Design review of the part built by this model. Coordinates are the model's own, in mm. Face numbers are marked on the shaded views. Give positions to 0.01 mm unless a question says otherwise; leave off trailing zeros. Write each loop counter-clockwise with the first axis right and the second up, starting at its lowest first coordinate (ties: lowest second). Pieces come first, ordered by that corner, then holes. Notation, with made-up numbers: M 63,4.5 L 113,4.5 A23 cw 113,22.5 Z; hole C 64.25,33 d2. An arc over 180 degrees is marked long. Use one line per item in the form item = value. Start each with the question number.
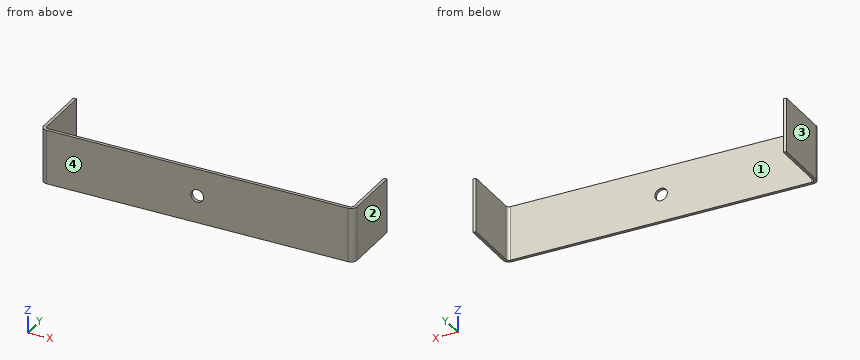
from build123d import *

# Parameters (mm, degrees)
SM_BASE_FLANGE_1_DEPTH = 6.5
OTHER_1_OUTLINE_R      = 1.5
OTHER_1_DEPTH          = 0.7366


# Read off the part's stored shape, not the designer's step: Отверстие1
# Sheet-metal steps are written as plain solids
with BuildPart() as part:
    # Sketch 1 → Базовая кромка1 (new, symmetric)
    with BuildSketch(Plane.XY):
        with BuildLine():
            Line((-37.5, 15), (-37.5, 1.4732))
            ThreePointArc((-37.5, 1.4732), (-37.06850971, 0.43149029), (-36.0268, 0))
            Line((-36.0268, 0), (36.0268, 0))
            ThreePointArc((36.0268, 0), (37.06850971, 0.43149029), (37.5, 1.4732))
            Line((37.5, 1.4732), (37.5, 15))
            Line((37.5, 15), (36.7634, 15))
            Line((36.7634, 15), (36.7634, 1.4732))
            ThreePointArc((36.7634, 1.4732), (36.547654855, 0.952345145), (36.0268, 0.7366))
            Line((36.0268, 0.7366), (-36.0268, 0.7366))
            ThreePointArc((-36.0268, 0.7366), (-36.547654855, 0.952345145), (-36.7634, 1.4732))
            Line((-36.7634, 1.4732), (-36.7634, 15))
            Line((-36.7634, 15), (-37.5, 15))
        make_face()
    extrude(amount=SM_BASE_FLANGE_1_DEPTH, both=True)

    # Отверстие1 outline → Отверстие1 (cut)
    with BuildSketch(Plane(origin=(0, 0, 0), x_dir=(1, 0, 0), z_dir=(0, 1, 0))):
        Circle(OTHER_1_OUTLINE_R)
    extrude(amount=OTHER_1_DEPTH, mode=Mode.SUBTRACT)


solid = part.part
1. Clearance check with flat-ended pins moving along their axes: pin 1 Ø8 at (x, y) = (10, 6) entering from -Z; pin 2 Ø4 at (x, z) = (0, 0) entering from +Y. State where each tip first meets the part, or that it passes through.
2. We need section B-B (y = 10.75). State the section outline as (x, z) points, and give its area (3 significant figures).
3. We need section A-A (x = 0). State the section outline as (y, z) points.
4. Draft analysis for pull direction X (two halves, no side actions). For the marked faces 1, 2, 3 and 4, state which applies: pulls with the +X half, pulls with the -X half, needs draft (parallel to the pull), parting line crosses it, or undercut.
5. We need section C-C (z = 0). State the section outline as (x, y) points.
6. We need section D-D (z = 4.5). State the section outline as (x, y) points, and give its area (3 significant figures).
7. To check wall thickness, follow L1, parallel to X at y = 1.5, z = 2.75; L2, parallel to Z at x = 0, y = 0.2; L3, parallel to X at y = 0.2, z = 0. State the ranges of each line that lie inside material, in increasing order.
Answer block:
q1.pin_1 = through
q1.pin_2 = 0.74
q2.outline = M -37.5,-6.5 L -36.76,-6.5 L -36.76,6.5 L -37.5,6.5 Z; M 36.76,-6.5 L 37.5,-6.5 L 37.5,6.5 L 36.76,6.5 Z
q2.area = 19.2 mm^2
q3.outline = M 0,-6.5 L 0.74,-6.5 L 0.74,-1.5 L 0,-1.5 Z; M 0,1.5 L 0.74,1.5 L 0.74,6.5 L 0,6.5 Z
q4.face_1 = undercut
q4.face_2 = pulls with the +X half
q4.face_3 = pulls with the -X half
q4.face_4 = needs draft
q5.outline = M -37.5,1.47 A1.47 ccw -36.03,0 L -1.5,0 L -1.5,0.74 L -36.03,0.74 A0.74 cw -36.76,1.47 L -36.76,15 L -37.5,15 Z; M 1.5,0 L 36.03,0 A1.47 ccw 37.5,1.47 L 37.5,15 L 36.76,15 L 36.76,1.47 A0.74 cw 36.03,0.74 L 1.5,0.74 Z
q6.outline = M -37.5,1.47 A1.47 ccw -36.03,0 L 36.03,0 A1.47 ccw 37.5,1.47 L 37.5,15 L 36.76,15 L 36.76,1.47 A0.74 cw 36.03,0.74 L -36.03,0.74 A0.74 cw -36.76,1.47 L -36.76,15 L -37.5,15 Z
q6.area = 75.6 mm^2
q7.L1 = -37.5 to -36.76, 36.76 to 37.5
q7.L2 = -6.5 to -1.5, 1.5 to 6.5
q7.L3 = -36.77 to -1.5, 1.5 to 36.77
